Autodesk Inventor part; units mm, degrees
ref_plane "YZ Plane" through (0, 0, 0) normal (1, 0, 0) x (0, 1, 0)
ref_plane "XZ Plane" through (0, 0, 0) normal (0, 1, 0) x (-1, 0, 0)
ref_plane "XY Plane" through (0, 0, 0) normal (0, 0, 1) x (1, 0, 0)
sketch "草圖1" plane through (0, 0, 0) normal (1, 0, 0) x (0, 1, 0)
  line L0 (0, 0) -> (24.2691, 25.2193)
  line L1 (24.2691, 25.2193) -> (24.2691, -25.2193)
  line L2 (24.2691, -25.2193) -> (0, 0)
  line L3 (0, 0) -> (24.2691, 0)
  circle A0 centre (24.2691, 25.2193) radius 6.15
  circle A1 centre (24.2691, -25.2193) radius 6.15
  circle A2 centre (0, 0) radius 6.15
  circle A3 centre (24.2691, 25.2193) radius 8.5
  circle A4 centre (24.2691, -25.2193) radius 8.5
  circle A5 centre (0, 0) radius 8.5
  line L4 (26.2691, 16.9579) -> (26.2691, -16.9579)
  line L5 (22.2691, 16.9579) -> (22.2691, -16.9579)
  line L6 (17.0995, 20.6534) -> (4.2873, 7.3395)
  line L7 (4.2873, -7.3395) -> (17.0995, -20.6534)
  line L8 (19.9817, 17.8798) -> (7.1695, 4.5659)
  line L9 (7.1695, -4.5659) -> (19.9817, -17.8798)
  line L10 (8.2614, 2) -> (24.2691, 2)
  line L11 (8.2614, -2) -> (24.2691, -2)
  point P0 (22.2691, 2)
  point P1 (22.2691, -2)
  dimension "d0" = 92.2
  dimension "d1" = 35
  dimension "d2" = 35
  dimension "d3" = 12.3
  dimension "d4" = 17
  dimension "d5" = 2
  dimension "d6" = 2
  dimension "d7" = 2
  dimension "d8" = 2
  dimension "d9" = 2
  dimension "d10" = 2
  dimension "d13" = 2
  dimension "d14" = 2
extrude "擠出1" add sketch "草圖1" along normal blind 6 contours A2 L2 A5 L0 | L0 A5 L3 A2 | A2 L3 A5 L2 | A5 L6 A3 L0 | L0 A3 L8 A5 | A5 L9 A4 L2 | L2 A4 L7 A5 | A5 L10 L5 L3 | L3 L5 L11 A5 | A3 L1 A0 L0 | L0 A0 L1 A3 | A4 L1 A1 L2 | L2 A1 L1 A4 | L5 L10 L1 L3 | L3 L1 L11 L5 | L1 A3 L4 A4 | L5 A3 L1 L10 | L11 L1 A4 L5
equation "\"d6\" = d5"
equation "\"d7\" = d5"
equation "\"d8\" = d5"
equation "\"d9\" = d5"
equation "\"d10\" = d5"
equation "\"d13\" = d5"
equation "\"d14\" = d5"
properties part number "TriangleLink_CBF" material "ABS 塑膠"
Verification items for the finished model (mm, model axes). A direction names the side the tool comes from. Round coordinates to 2 decimals unless told otherwise and drop trailing zeros. Order: outer loops, then holes, each group sorted by start corner. A loop starts at its lowest first (then second) coordinate and runs counter-clockwise, first axis right, second up. Notation, with made-up numbers: (59, -17) - (92, -17) arc R13 ccw to (92, 4) - close; hole circle Ø1 at (45.25, 27.5). An arc over 180 degrees is marked (long way). Use CSV: the item, a comma, the result in double quotes.
(1) Section check B-B on z = 0. Record the boundary of the cut face in (x, y), and give its area (3 significant figures).
Entries:
outline,"(0, -8.5) - (6, -8.5) - (6, -6.15) - (0, -6.15) - close; (0, 6.15) - (6, 6.15) - (6, 26.27) - (0, 26.27) - close"
area,"135 mm^2"
(2) Section check C-C on x = 3.65. Record the boundary of the cut face in (y, z), and give its area (3 significant figures).
Entries:
outline,"(4.29, -7.34) - (17.1, -20.65) arc R8.5 ccw (long way) to (26.27, -16.96) - (26.27, 16.96) arc R8.5 ccw (long way) to (17.1, 20.65) - (4.29, 7.34) arc R8.5 ccw (long way) to start; hole circle Ø12.3 at (0, 0); hole (7.17, -4.57) - (19.98, -17.88) arc R8.5 cw to (22.27, -16.96) - (22.27, -2) - (8.26, -2) arc R8.5 cw to start; hole (7.17, 4.57) arc R8.5 cw to (8.26, 2) - (22.27, 2) - (22.27, 16.96) arc R8.5 cw to (19.98, 17.88) - close; hole circle Ø12.3 at (24.27, -25.22); hole circle Ø12.3 at (24.27, 25.22)"
area,"660 mm^2"
(3) Gauge pin test, flat ends, axial feed: pin 1 Ø1.8 at (x, y) = (4.5, 14) entering from +Z; pin 2 Ø3 at (x, z) = (3.5, -13.5) entering from +Y; pin 3 Ø3 at (x, y) = (4.5, 15.5) entering from +Z (3 decimals). Record the tip position at first contact, or that the pin passes through.
Entries:
pin 1,"z = 18.37"
pin 2,"y = 26.27"
pin 3,"z = 29.625"
(4) Mould release check, pull along Y, two halves, no side actions. Record for faces 4 (the face through (6, 17, 0)), 5 (the face through (3, 22.269, -9)), 6 (the face through (2.958, 27.723, -32.986)): released by +Y, released by -Y, zero draft, split by the parting line, or undercut.
Entries:
face 4,"zero draft"
face 5,"undercut"
face 6,"split by the parting line"
(5) Thickness scan on probe 1 along Z at (x, y) = (1.9, 0); probe 2 along Z at (x, y) = (3.8, 12); probe 3 along Z at (x, y) = (5.55, 14.5). Record the ranges inside material, lowest first. Write a range as from..to.
Entries:
probe 1,"-8.5..-6.15, 6.15..8.5"
probe 2,"-15.35..-9.59, -2..2, 9.59..15.35"
probe 3,"-17.95..-12.18, -2..2, 12.18..17.95"
(6) Access from +Z, -Z, +X, -X, +Y, -Y to the whole of each face (thin tool, end or side, straight path). Record for faces 1 (the face through (2.958, 13.486, -11.13)), 2 (the face through (0, 17, 0)), 3 (the face through (3, 26.269, 0)).
Entries:
face 1,"+X, -X"
face 2,"+Z, -Z, -X, +Y, -Y"
face 3,"+X, -X, +Y"
(7) Section check A-A on y = 0. Record the boundary of the cut face in (x, z).
Entries:
outline,"(0, -8.5) - (6, -8.5) - (6, -6.15) - (0, -6.15) - close; (0, 6.15) - (6, 6.15) - (6, 8.5) - (0, 8.5) - close"
